from build123d import *

# Parameters (mm, degrees)
CUT_EXTRUDE_1_DEPTH = 3


with BuildPart() as part:
    # Sketch 1 → Revolve 1 (revolve)
    with BuildSketch(Plane.XY, mode=Mode.PRIVATE) as revolve_1_sk:
        Polygon((-5, 0), (-5, 2.4), (-0.5, 2.4), (-0.5, 1.5), (0, 1.5), (0, 2.4585), (0.5415, 3), (24.4585, 3), (25, 2.4585), (25, 0), align=None)
    revolve(revolve_1_sk.sketch.rotate(Axis((25, 0, 0), (-1, 0, 0)), 270), axis=Axis((25, 0, 0), (-1, 0, 0)))

    # Sketch 2 → Cut-Revolve 1 (revolve, cut)
    with BuildSketch(Plane(origin=(0, 0, 0), x_dir=(1, 0, 0), z_dir=(0, 1, 0)), mode=Mode.PRIVATE) as cut_revolve_1_sk:
        Polygon((21.133974596, 0), (22, 1.5), (25, 1.5), (25, 0), align=None)
    revolve(cut_revolve_1_sk.sketch.rotate(Axis((25, 0, 0), (-1, 0, 0)), 180), axis=Axis((25, 0, 0), (-1, 0, 0)), mode=Mode.SUBTRACT)

    # Sketch 3 → Cut-Extrude 1 (cut)
    with BuildSketch(Plane(origin=(25, 0, 0), x_dir=(0, 0, -1), z_dir=(1, 0, 0))):
        Polygon((-1.5, 0.866025404), (-1.5, -0.866025404), (0, -1.732050808), (1.5, -0.866025404), (1.5, 0.866025404), (0, 1.732050808), align=None)
    extrude(amount=-CUT_EXTRUDE_1_DEPTH, mode=Mode.SUBTRACT)


solid = part.part
Check sheet for the modelled part. Datum: model origin and axes. Units: mm. A direction names the side the tool comes from. Give positions to 0.01 mm unless a question says otherwise; leave off trailing zeros. Write each loop counter-clockwise with the first axis right and the second up, starting at its lowest first coordinate (ties: lowest second). Pieces come first, ordered by that corner, then holes. Notation, with made-up numbers: (-23.5, 10.5) -> (26.5, 10.5) arc R31 ccw to (26.5, 49.5) -> close; hole circle Ø4 at (63.25, 60). An arc over 180 degrees is marked (long way). One line per item, written item: value. Start each with the question number.
Item 1: Material ranges on probe 1 along X at (y, z) = (-0.3, -1.75); probe 2 along Y at (x, z) = (19, -2.6); probe 3 along Y at (x, z) = (-2, 0.05), recorded low to high. Write a range as from..to.
Item 2: Draft check along X on faces 4 (the flat face through (-5, 0, 0)), 5 (the cylindrical face through (-0.25, 0.45, 1.43)), 6 (the conical face through (21.284, -0.231, 0.12)), 7 (the cylindrical face through (12.67, 0.9, 2.86)). Enter one of: +X half, -X half, draft (parallel to the pull), parting line (faces both ways), or undercut.
Item 3: Tool access check on faces 1 (the flat face through (23.521, -1.305, -0.74)), 2 (the cylindrical face through (-2.718, 2.024, 1.29)), 3 (the flat face through (0, -2, 0)). Record the directions out of +Z, -Z, +X, -X, +Y, -Y that give a thin tool (end or side, any length) a straight path to the whole face; none if there is none.
Item 4: Section check A-A on x = -2.5. Record the cut outline in (y, z), then the cut area to 3 significant figures.
Item 5: Gauge pin test, flat ends, axial feed: pin 1 (0.6 mm diameter, centred on y = 0.5, z = 1, fed in from +X); pin 2 (0.5 mm diameter, centred on x = 23.5, y = 0.5, fed in from +Z); pin 3 (1 mm diameter, centred on x = 20.5, y = 1, fed in from -Z). Record the tip position at first contact, or that the pin passes through.
Item 6: Section check B-B on x = 16.25. Record the cut outline in (y, z), then the cut area to 3 significant figures.
Results list:
1. probe 1: -5..-0.5, 0..25
1. probe 2: -1.5..1.5
1. probe 3: -2.4..2.4
2. face 4: -X half
2. face 5: undercut
2. face 6: +X half
2. face 7: draft
3. face 1: +X
3. face 2: -X
3. face 3: none
4. outline: circle Ø4.8 at (0, 0)
4. area: 18.1 mm²
5. pin 1: x = 21.95
5. pin 2: z = 2.99
5. pin 3: z = -2.96
6. outline: circle Ø6 at (0, 0)
6. area: 28.3 mm²
